```python
from build123d import *

# Parameters (mm, degrees)
SKETCH1_R           = 11
BOSS_EXTRUDE1_DEPTH = 3
BOSS_EXTRUDE2_DEPTH = 3
SKETCH3_R           = 11
BOSS_EXTRUDE3_DEPTH = 3
SKETCH4_R           = 5
CUT_EXTRUDE1_DEPTH  = 10
SKETCH5_R           = 1
CUT_EXTRUDE2_DEPTH  = 3


with BuildPart() as part:
    # Sketch1 → Boss-Extrude1 (new body)
    with BuildSketch(Plane.XY):
        Circle(SKETCH1_R)
    extrude(amount=BOSS_EXTRUDE1_DEPTH)

    # Sketch2 → Boss-Extrude2 (add)
    with BuildSketch(Plane.XY.offset(3)):
        with BuildLine():
            Line((-11, 0), (-9.5, 11))
            Line((-9.5, 11), (9.5, 11))
            Line((9.5, 11), (11, 0))
            ThreePointArc((11, 0), (0, -11), (-11, 0))
        make_face()
    extrude(amount=BOSS_EXTRUDE2_DEPTH)

    # Sketch3 → Boss-Extrude3 (add)
    with BuildSketch(Plane.XY.offset(6)):
        Circle(SKETCH3_R)
    extrude(amount=BOSS_EXTRUDE3_DEPTH)

    # Sketch4 → Cut-Extrude1 (cut, through all)
    with BuildSketch(Plane.XY.offset(9)):
        Circle(SKETCH4_R)
    extrude(amount=-CUT_EXTRUDE1_DEPTH, mode=Mode.SUBTRACT)

    # Sketch5 → Cut-Extrude2 (cut)
    with BuildSketch(Plane(origin=(0, 11, 0), x_dir=(1, 0, 0), z_dir=(0, 1, 0))):
        with Locations((-6.5, -4.5)):
            Circle(SKETCH5_R)
        with Locations((6.5, -4.5)):
            Circle(SKETCH5_R)
    extrude(amount=-CUT_EXTRUDE2_DEPTH, mode=Mode.SUBTRACT)


solid = part.part
```
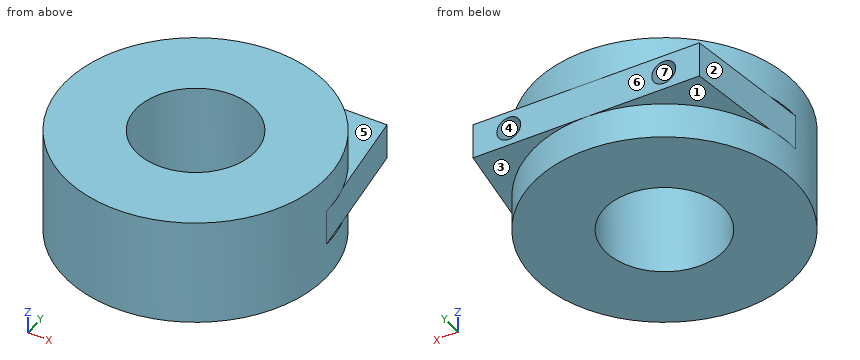
The model under review builds one solid part; all positions refer to its coordinate system, in mm. Face numbers are marked on the shaded views. A direction names the side the tool comes from. Coordinates: 2 decimals unless noted, no trailing zeros. Order: outer loops, then holes, each group sorted by start corner. A loop starts at its lowest first (then second) coordinate and runs counter-clockwise, first axis right, second up. Notation, with made-up numbers: (76.25, -2.75) -> (80.25, -2.75) arc R16 ccw to (80.25, 5.25) -> close; hole circle Ø4 at (51, -28.75). An arc over 180 degrees is marked (long way). Answer in a Markdown table with one row per item. Add a question column.
Item 1: To check wall thickness, follow probe 1 along Z at (x, y) = (6.5, 9.25); probe 2 along X at (y, z) = (9.45, 4.5); probe 3 along X at (y, z) = (2.5, 1.25). State the ranges of each line that lie inside material, in increasing order.
Item 2: We need section C-C on x = 3.5. Write out the cut boundary in (y, z).
Item 3: Machinability: for the marked faces 1, 2, 3 and 4, which of the approach directions +Z, -Z, +X, -X, +Y, -Y give a long, thin tool a straight path to every point of the face, cutting with its end or side? Answer none if there is none.
Item 4: Clearance check with flat-ended pins moving along their axes: pin 1 (3 mm diameter, centred on x = -6.5, z = 4.5, fed in from -Y); pin 2 (4 mm diameter, centred on x = -3, y = 1.5, fed in from -Z); pin 3 (0.6 mm diameter, centred on x = -6.5, z = 5, fed in from +Y). State where each tip first meets the part, or that it passes through.
Item 5: Mouldability with a two-part tool opening along Z and no side actions: class the marked faces 5, 6 and 7 as +Z half, -Z half, draft (parallel to the pull), parting line (faces both ways), or undercut.
Item 6: We need section B-B on y = 8.5. Write out the cut boundary in (x, z), plus the area to 3 significant figures.
Item 7: We need section A-A on z = 4.5. Write out the cut boundary in (x, y), plus the area to 3 significant figures.
Item 8: We need section D-D on y = -3. Write out the cut boundary in (x, z).
Final values:
| question | item | result |
|---|---|---|
| 1 | probe 1 | z = 3 to 3.5, 5.5 to 6 |
| 1 | probe 2 | x = -9.71 to -7.5, -5.5 to 5.5, 7.5 to 9.71 |
| 1 | probe 3 | x = -10.71 to -4.33, 4.33 to 10.71 |
| 2 | outline | (-10.43, 0) -> (-3.57, 0) -> (-3.57, 9) -> (-10.43, 9) -> close; (3.57, 0) -> (10.43, 0) -> (10.43, 3) -> (11, 3) -> (11, 6) -> (10.43, 6) -> (10.43, 9) -> (3.57, 9) -> close |
| 3 | face 1 | -Z, -X, +Y |
| 3 | face 2 | -X, +Y |
| 3 | face 3 | -Z, +X, +Y |
| 3 | face 4 | +Y |
| 4 | pin 1 | stops at y = -9.8 |
| 4 | pin 2 | stops at z = 0 |
| 4 | pin 3 | stops at y = 8 |
| 5 | face 5 | +Z half |
| 5 | face 6 | draft |
| 5 | face 7 | undercut |
| 6 | outline | (-9.84, 3) -> (-6.98, 3) -> (-6.98, 0) -> (6.98, 0) -> (6.98, 3) -> (9.84, 3) -> (9.84, 6) -> (6.98, 6) -> (6.98, 9) -> (-6.98, 9) -> (-6.98, 6) -> (-9.84, 6) -> close; hole circle Ø2 at (-6.5, 4.5); hole circle Ø2 at (6.5, 4.5) |
| 6 | area | 137 mm2 |
| 7 | outline | (-11, 0) arc R11 ccw to (11, 0) -> (9.5, 11) -> (7.5, 11) -> (7.5, 8) -> (5.5, 8) -> (5.5, 11) -> (-5.5, 11) -> (-5.5, 8) -> (-7.5, 8) -> (-7.5, 11) -> (-9.5, 11) -> close; hole circle Ø10 at (0, 0) |
| 7 | area | 325 mm2 |
| 8 | outline | (-10.58, 0) -> (-4, 0) -> (-4, 9) -> (-10.58, 9) -> close; (4, 0) -> (10.58, 0) -> (10.58, 9) -> (4, 9) -> close |
